Work out the finished part from the listing and answer in its coordinate system (mm). Round coordinates to 2 decimals unless told otherwise and drop trailing zeros. Order: outer loops, then holes, each group sorted by start corner. A loop starts at its lowest first (then second) coordinate and runs counter-clockwise, first axis right, second up. Notation, with made-up numbers: M 52,68.5 L 74,68.5 A11 cw 74,81.5 Z; hole C -8.75,21.5 d4. An arc over 180 degrees is marked long. Answer as a JSON object with one key per item and string values. Group by question number.
Autodesk Inventor part; units mm, degrees
ref_plane "YZ Plane" through (0, 0, 0) normal (1, 0, 0) x (0, 1, 0)
ref_plane "XZ Plane" through (0, 0, 0) normal (0, 1, 0) x (-1, 0, 0)
ref_plane "XY Plane" through (0, 0, 0) normal (0, 0, 1) x (1, 0, 0)
sketch "Sketch1" plane through (0, 0, 0) normal (0, 0, 1) x (1, 0, 0)
  line L0 (0, 0) -> (38.1, 0)
  line L1 (38.1, 0) -> (38.1, -30.48)
  line L2 (38.1, -30.48) -> (0, -30.48)
  line L3 (0, -30.48) -> (0, 0)
  circle A0 centre (6.35, -15.24) radius 1.5875
  circle A1 centre (31.75, -15.24) radius 1.5875
  dimension "d0" = 38.1
  dimension "d1" = 30.48
  dimension "d2" = 6.35
  dimension "d3" = 6.35
  dimension "d4" = 3.175
  dimension "d5" = 3.175
extrude "Extrusion1" add sketch "Sketch1" along normal blind 3.175
properties part number "Plate" material "Aluminum 6061"
Item 1: This flat-tipped pin is pushed along its axis until it touches: pin 1 (3 mm diameter, centred on x = 6.35, y = -15.24, fed in from -Z). Where does it stop, or does it pass through?
Item 2: Find section A-A (y = -15.24). Give the vertices of the cut face in (x, z) (1 decimal).
Item 3: Consider L1, parallel to Y at x = 6.35, z = 2.35; L2, parallel to X at y = -15.5, z = 1.4; L3, parallel to Y at x = 31, z = 2.65. Determine where each line is inside the solid, lowest interval first.
Item 4: The mould has two halves that part along X. Classify faces 1 (the flat face through (0, -15, 2)), 2 (the cylindrical face through (33.264, -15.717, 1.565)), 3 (the flat face through (19, -15, 3.175)): +X half, -X half, draft (parallel to the pull), parting line (faces both ways), or undercut.
Item 5: Find section B-B (x = 31.75). Give the vertices of the cut face in (y, z) (1 decimal).
Item 6: Find section C-C (x = 7.5). Give the vertices of the cut face in (y, z) (3 decimals), and give its area (3 significant figures).
Responses:
{
 "1": {"pin 1": "passes through"},
 "2": {"outline": "M 0,0 L 4.8,0 L 4.8,3.2 L 0,3.2 Z; M 7.9,0 L 30.2,0 L 30.2,3.2 L 7.9,3.2 Z; M 33.3,0 L 38.1,0 L 38.1,3.2 L 33.3,3.2 Z"},
 "3": {"L1": "y = -30.48 to -16.83, -13.65 to 0", "L2": "x = 0 to 4.78, 7.92 to 30.18, 33.32 to 38.1", "L3": "y = -30.48 to -16.64, -13.84 to 0"},
 "4": {"face 1": "-X half", "face 2": "undercut", "face 3": "draft"},
 "5": {"outline": "M -30.5,0 L -16.8,0 L -16.8,3.2 L -30.5,3.2 Z; M -13.7,0 L 0,0 L 0,3.2 L -13.7,3.2 Z"},
 "6": {"outline": "M -30.48,0 L -16.334,0 L -16.334,3.175 L -30.48,3.175 Z; M -14.146,0 L 0,0 L 0,3.175 L -14.146,3.175 Z", "area": "89.8 mm^2"}
}
